Source: CAD feature listing. Evaluate the final solid. Frame: model axes, mm. A direction names the side the tool comes from. Give positions to 0.01 mm unless a question says otherwise; leave off trailing zeros. Order: outer loops, then holes, each group sorted by start corner. A loop starts at its lowest first (then second) coordinate and runs counter-clockwise, first axis right, second up. Notation, with made-up numbers: M 52,28.5 L 61,28.5 A11 ccw 61,34.5 Z; hole C 18,17 d11. An arc over 180 degrees is marked long. Answer in a Markdown table with one row per item. Add a question column.
(1) Mould query, pull axis Z, two halves, no side actions, for faces 6 (the face through (-21.4, -0.1, 34.2)), 7 (the face through (47.69, 15.02, 2.46)), 8 (the face through (-21.585, -0.14, 15)). Classes: pulls with the +Z half, pulls with the -Z half, needs draft (parallel to the pull), parting line crosses it, or undercut.
(2) Set-up query: faces 1 (the face through (-1, 1, 0)), 2 (the face through (-36.47, -0.14, 15.21)), 3 (the face through (-39, 0, 43.29)), 4 (the face through (-26, -10, 24)), 5 (the face through (-26, 10, 24)). Return all of +Z, -Z, +X, -X, +Y, -Y with unobstructed straight access to the full face (end or side cutting, diameter ignored); none if empty.
(3) Section query A-A, the plane y = 0. Return loops of the section in (x, z).
(4) Pin query (flat end, axial travel): P1, Ø2, axis at x = -21.5, y = -36.5, coming from the +Z side; P2, Ø10.5, axis at x = -34, z = 30, coming from the +Y side; P3, Ø10, axis at x = -7, y = -34, coming from the -Z side; P4, Ø10.5, axis at x = -29.5, z = 33.5, coming from the -Y side. Return the tip coordinate at first contact, or that it passes through.
(5) Section query C-C, the plane z = 38. Return loops of the section in (x, y).
(6) Section query B-B, the plane x = 0. Return loops of the section in (y, z).
(7) Material intervals for line 1 along Y through (x, z) = (-36, 6.5); line 2 along Z through (x, y) = (14.5, 1.5); line 3 along X through (y, z) = (-38, 4), sorted ascending.
from build123d import *

# Parameters (mm, degrees)
F2_R     = 50
F3_DEPTH = 5
F6_DEPTH = 10


with BuildPart() as f3:
    # F2 (on face) → F3 (new body)
    with BuildSketch(Plane.XY):
        Circle(F2_R)
    extrude(amount=F3_DEPTH)

    # F5 (on face) → F6 (join, symmetric)
    with BuildSketch(Plane.XZ):
        Polygon((-46.88603, 43.289871), (-27.134711, 25.138109), (-46.067975, 5), (-30.987105, 5), (-11.916471, 25.284221), (-31.067937, 43.289871), align=None)
    extrude(amount=F6_DEPTH, both=True)


solid = f3.part
Values follow:
| question | item | result |
|---|---|---|
| 1 | face 6 | pulls with the +Z half |
| 1 | face 7 | needs draft |
| 1 | face 8 | undercut |
| 2 | face 1 | -Z, +X, -X, +Y, -Y |
| 2 | face 2 | -X, +Y, -Y |
| 2 | face 3 | +Z, +X, -X, +Y, -Y |
| 2 | face 4 | +Z, +X, -X, -Y |
| 2 | face 5 | +Z, +X, -X, +Y |
| 3 | outline | M -50,0 L 50,0 L 50,5 L -30.99,5 L -11.92,25.28 L -31.07,43.29 L -46.89,43.29 L -27.13,25.14 L -46.07,5 L -50,5 Z |
| 4 | P1 | stops at z = 5 |
| 4 | P2 | stops at y = 10 |
| 4 | P3 | stops at z = 0 |
| 4 | P4 | stops at y = -10 |
| 5 | outline | M -41.13,-10 L -25.44,-10 L -25.44,10 L -41.13,10 Z |
| 6 | outline | M -50,0 L 50,0 L 50,5 L -50,5 Z |
| 7 | line 1 | y = -10 to 10 |
| 7 | line 2 | z = 0 to 5 |
| 7 | line 3 | x = -32.5 to 32.5 |
